from build123d import *

# Parameters (mm, degrees)
F1_DEPTH = 63.5
F2_DEPTH = 25.4
F3_DEPTH = 7.9375
F5_R     = 38.1


with BuildPart() as f1:
    # F0 (on Front) → F1 (new body, symmetric)
    with BuildSketch(Plane.XZ):
        Polygon((41.275, 9.525), (27.305, 9.525), (-41.1475321427, 9.525), (-41.275, 9.525), (-41.275, -9.525), (41.275, -9.525), align=None)
    extrude(amount=F1_DEPTH, both=True)

    # F0 (on Front) → F2 (join, symmetric)
    with BuildSketch(Plane.XZ):
        with BuildLine():
            Line((27.305, 50.2448773877), (27.305, 9.525))
            Line((27.305, 9.525), (41.275, 9.525))
            Line((41.275, 9.525), (41.275, 50.2448773877))
            ThreePointArc((41.275, 50.2448773877), (45.9090266229, 60.6372063424), (56.7367753904, 64.135))
            Line((56.7367753904, 64.135), (60.325, 64.135))
            Line((60.325, 64.135), (60.325, 78.105))
            Line((60.325, 78.105), (57.3562006129, 78.105))
            add(Edge.make_bspline(
                [(52.937874551, 78.0894598439), (54.3919964318, 78.1126841505), (55.864731429, 78.1180111613), (57.3562006129, 78.105)],
                knots=[117.4190282855, 117.4190282855, 117.4190282855, 117.4190282855, 120.108518673, 120.108518673, 120.108518673, 120.108518673], degree=3))
            ThreePointArc((52.937874551, 78.0894598439), (34.6889220053, 69.1681767162), (27.305, 50.2448773877))
        make_face()
        Polygon((60.325, 78.105), (60.325, 64.135), (85.725, 64.135), (85.725, 71.4375), (85.725, 78.105), align=None)
    extrude(amount=F2_DEPTH, both=True)

    # F0 (on Front) → F3 (join, symmetric)
    with BuildSketch(Plane.XZ):
        with BuildLine():
            Line((-41.1475321427, 9.525), (27.305, 9.525))
            Line((27.305, 9.525), (27.305, 50.2448773877))
            ThreePointArc((27.305, 50.2448773877), (34.6889220053, 69.1681767162), (52.937874551, 78.0894598439))
            add(Edge.make_bspline(
                [(-41.1475321427, 9.525), (-38.4794783387, 42.0413634319), (-10.4626480253, 77.0768671657), (52.937874551, 78.0894598439)],
                knots=[0.1557518826, 0.1557518826, 0.1557518826, 0.1557518826, 117.4190282855, 117.4190282855, 117.4190282855, 117.4190282855], degree=3))
        make_face()
    extrude(amount=F3_DEPTH, both=True)

    # F0 (on Front) → F4 (revolve)
    with BuildSketch(Plane.XZ):
        Polygon((85.725, 71.4375), (85.725, 64.135), (85.725, 57.15), (111.125, 57.15), (111.125, 85.725), (85.725, 85.725), (85.725, 78.105), align=None)
    revolve(axis=Axis((85.725, 0, 71.4375), (0, 0, 1)))

    # F5
    f5_edges = [f1.edges().sort_by_distance(p)[0] for p in [
        (-41.275, -63.5, 0),
        (41.275, -63.5, 0),
        (41.275, 63.5, 0),
        (-41.275, 63.5, 0),
    ]]
    fillet(f5_edges, radius=F5_R)


solid = f1.part
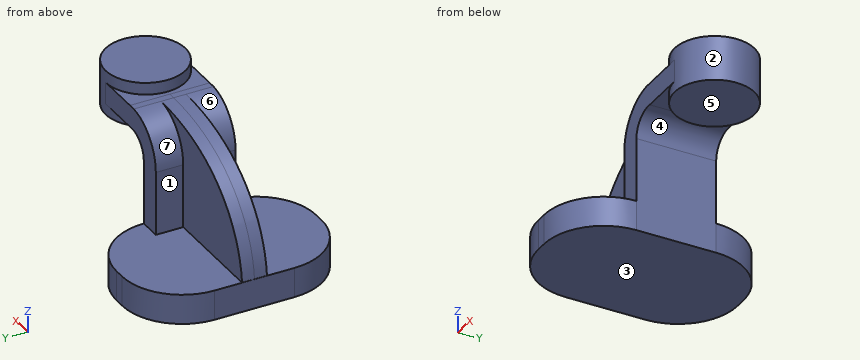
Verification items for the finished model (mm, model axes). Face numbers are marked on the shaded views. A direction names the side the tool comes from. Round coordinates to 2 decimals unless told otherwise and drop trailing zeros. Loops run counter-clockwise (first coordinate to the right, second up) from the corner with the lowest first, then second, coordinate; pieces in that order, holes last. Notation, with made-up numbers: M 61.5,69 L 115.5,69 A14 ccw 115.5,90 Z; hole C 60,60 d2. An arc over 180 degrees is marked long. Write each question's results on one line, items separated by ' | '.
1) Section check B-B on y = 49. Record the boundary of the cut face in (x, z) (3 decimals).
Checks:
outline: M -33.086,-9.525 L 33.086,-9.525 L 33.086,9.525 L -33.086,9.525 Z
2) Section check A-A on x = 71. Record the boundary of the cut face in (y, z) (3 decimals), then the cut area to 3 significant figures.
Checks:
outline: M -25.4,64.135 L -20.696,64.135 L -20.696,57.15 L 20.696,57.15 L 20.696,64.135 L 25.4,64.135 L 25.4,78.105 L 20.696,78.105 L 20.696,85.725 L -20.696,85.725 L -20.696,78.105 L -25.4,78.105 Z | area: 1,310 mm2
3) Mould release check, pull along X, two halves, no side actions. Record for the marked faces 1, 2, 3 and 4: released by +X, released by -X, zero draft, split by the parting line, or undercut.
Checks:
face 1: released by -X | face 2: undercut | face 3: zero draft | face 4: undercut
4) Section check C-C on y = -43.5. Record the boundary of the cut face in (x, z) (3 decimals), then the cut area to 3 significant figures.
Checks:
outline: M -36.701,-9.525 L 36.701,-9.525 L 36.701,9.525 L -36.701,9.525 Z | area: 1,400 mm2
5) Scan lines: L1, parallel to X at y = 11.5, z = -2 (3 decimals); L2, parallel to Z at x = 18, y = -41.5 (3 decimals); L3, parallel to Z at x = 57.5, y = 10 (3 decimals). Record each from-to range of solid material in increasing order. Write a range as from..to.
Checks:
L1: x = -41.275..41.275 | L2: z = -9.525..9.525 | L3: z = 64.135..78.105
6) Gauge pin test, flat ends, axial feed: P1, Ø8.5, axis at x = 78, y = 7.5, coming from the -Z side; P2, Ø4, axis at y = -28.5, z = 66.5, coming from the +X side; P3, Ø8.5, axis at y = -16, z = 29, coming from the -X side (3 decimals); P4, Ø6, axis at x = -6.5, z = 4, coming from the -Y side. Record the tip position at first contact, or that the pin passes through.
Checks:
P1: stops at z = 57.15 | P2: passes through | P3: stops at x = 27.305 | P4: stops at y = -63.5
7) Access from +Z, -Z, +X, -X, +Y, -Y to the whole of each face (thin tool, end or side, straight path). Record for the marked faces 5, 6 and 7.
Checks:
face 5: -Z, +X, +Y, -Y | face 6: +Z, -X, -Y | face 7: +Z, -X, +Y
